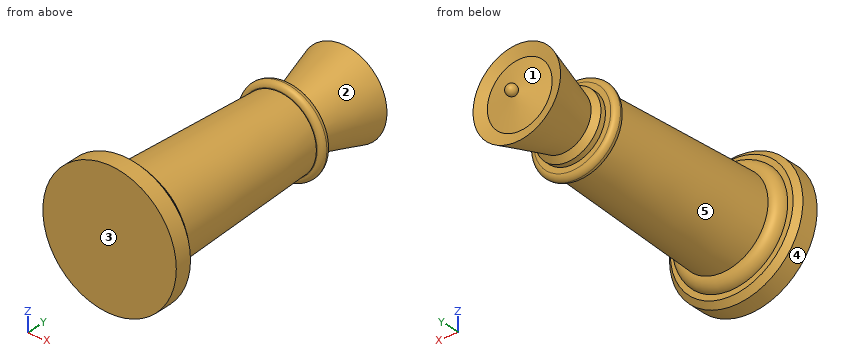
```python
from build123d import *

# Parameters (mm, degrees)
CHAMFER1_SIZE = 0.03
FILLET1_R     = 0.06
FILLET2_R     = 0.03


# Read off the part's stored shape, not the designer's step: Scale1
with BuildPart() as part:
    # Sketch1 → Revolve1 (revolve)
    with BuildSketch(Plane.XY, mode=Mode.PRIVATE) as revolve1_sk:
        with BuildLine():
            Line((0, 0), (-0.375, 0))
            Line((-0.375, 0), (-0.375, 0.125))
            Line((-0.375, 0.125), (-0.315, 0.125))
            Line((-0.315, 0.125), (-0.315, 0.185))
            Line((-0.315, 0.185), (-0.255, 0.185))
            Line((-0.255, 0.185), (-0.212, 1.129))
            Line((-0.212, 1.129), (-0.246, 1.129))
            Line((-0.246, 1.129), (-0.246, 1.189))
            Line((-0.246, 1.189), (-0.186, 1.189))
            Line((-0.186, 1.189), (-0.186, 1.249))
            Line((-0.186, 1.249), (-0.156, 1.249))
            Line((-0.156, 1.249), (-0.246, 1.56))
            Line((-0.246, 1.56), (-0.182, 1.54))
            Line((-0.182, 1.54), (-0.022424467, 1.575071546))
            ThreePointArc((-0.022424467, 1.575071546), (-0.027366527, 1.607291183), (0, 1.625))
            Line((0, 1.625), (0, 0))
        make_face()
    revolve(revolve1_sk.sketch.rotate(Axis((0, 0, 0), (0, 1, 0)), 270), axis=Axis((0, 0, 0), (0, 1, 0)))

    # Chamfer1
    chamfer1_edges = [part.edges().sort_by_distance(p)[0] for p in [
        (0, 0.125, 0.375),
        (0, 1.249, 0.186),
    ]]
    chamfer(chamfer1_edges, length=CHAMFER1_SIZE - 0.0001)  # a hair under: the kernel refuses the full size

    # Fillet1
    fillet1_edges = [part.edges().sort_by_distance(p)[0] for p in [
        (0, 0.185, 0.315),
    ]]
    fillet(fillet1_edges, radius=FILLET1_R - 0.0001)  # a hair under: the kernel refuses the full size

    # Fillet2
    fillet2_edges = [part.edges().sort_by_distance(p)[0] for p in [
        (0, 1.129, 0.246),
        (0, 1.189, 0.246),
    ]]
    fillet(fillet2_edges, radius=FILLET2_R - 0.0001)  # a hair under: the kernel refuses the full size

    # Scale1 outline → Scale1 (revolve)
    with BuildSketch(Plane.XY):
        with BuildLine():
            Line((5.46, 27.865595941), (0.672734004, 28.917742313))
            ThreePointArc((0.672734004, 28.917742313), (0.820995818, 29.884331439), (0, 30.415595941))
            Line((0, 30.415595941), (0, 1.625))
            ThreePointArc((0, 1.625), (0.027366527, 1.607291183), (0.022424467, 1.575071546))
            Line((0.022424467, 1.575071546), (0.182, 1.54))
            Line((0.182, 1.54), (0.246, 1.56))
            Line((0.246, 1.56), (0.156, 1.249))
            Line((0.156, 1.249), (0.186, 1.219))
            Line((0.186, 1.219), (0.186, 1.189))
            Line((0.186, 1.189), (0.216, 1.189))
            ThreePointArc((0.216, 1.189), (0.237213203, 1.180213203), (0.246, 1.159))
            ThreePointArc((0.246, 1.159), (0.237213203, 1.137786797), (0.216, 1.129))
            Line((0.216, 1.129), (0.212, 1.129))
            Line((0.212, 1.129), (0.255, 0.185))
            ThreePointArc((0.255, 0.185), (0.297426407, 0.167426407), (0.315, 0.125))
            Line((0.315, 0.125), (0.345, 0.125))
            Line((0.345, 0.125), (0.375, 0.095))
            Line((0.375, 0.095), (0.375, 0))
            Line((0.375, 0), (0, 0))
            Line((0, 0), (0, -18.334404059))
            Line((0, -18.334404059), (11.25, -18.334404059))
            Line((11.25, -18.334404059), (11.25, -15.484404059))
            Line((11.25, -15.484404059), (10.35, -14.584404059))
            Line((10.35, -14.584404059), (9.45, -14.584404059))
            ThreePointArc((9.45, -14.584404059), (8.922792206, -13.311611853), (7.65, -12.784404059))
            Line((7.65, -12.784404059), (6.36, 15.535595941))
            Line((6.36, 15.535595941), (6.48, 15.535595941))
            ThreePointArc((6.48, 15.535595941), (7.116396103, 15.799199838), (7.38, 16.435595941))
            ThreePointArc((7.38, 16.435595941), (7.116396103, 17.071992044), (6.48, 17.335595941))
            Line((6.48, 17.335595941), (5.58, 17.335595941))
            Line((5.58, 17.335595941), (5.58, 18.235595941))
            Line((5.58, 18.235595941), (4.68, 19.135595941))
            Line((4.68, 19.135595941), (7.38, 28.465595941))
            Line((7.38, 28.465595941), (5.46, 27.865595941))
        make_face()
    revolve(axis=Axis((0, 0, 0), (0, 1, 0)))


solid = part.part
```
Here's how the part is built. I have some questions about the finished solid (model axes, mm). Face numbers are marked on the shaded views. A direction names the side the tool comes from. Give positions to 0.01 mm unless a question says otherwise; leave off trailing zeros. Order: outer loops, then holes, each group sorted by start corner. A loop starts at its lowest first (then second) coordinate and runs counter-clockwise, first axis right, second up. Notation, with made-up numbers: (71, 8.5) -> (81, 8.5) arc R24 ccw to (81, 46.5) -> close; hole circle Ø5 at (-40, 6). An arc over 180 degrees is marked (long way). Use CSV: the item, a comma, the result in double quotes. Start each with the question number.
Item 1: If I drill on probe 1 along Y at (x, z) = (9.25, 3.5); probe 2 along X at (y, z) = (-0.5, -5); probe 3 along X at (y, z) = (14, -2), over which ranges is the centre line in solid material (lowest first)? Write a range as [from, to].
Item 2: Thinking about a two-plate mould opening in X: for the marked faces 1, 2 and 3, which applies, pulls with the +X half, pulls with the -X half, needs draft (parallel to the pull), parting line crosses it, or undercut?
Item 3: On a 3-axis mill with a long thin cutter (end or side, diameter ignored), from which of +Z, -Z, +X, -X, +Y, -Y can I reach the whole of each face in a straight line? I mean the marked faces 4 and 5. Say none if no direction works.
Item 4: I'm going to push flat-ended pins straight in: P1, Ø4, axis at x = -2.5, z = -2, coming from the +Y side; P2, Ø10, axis at x = 6.5, z = -2.5, coming from the +Y side; P3, Ø1.5, axis at x = 1, y = 9, coming from the +Z side. Where does each tip first touch, or does it pass through?
Item 5: Suppose I cut it at A-A (y = 8). List the corners of the cut face in (x, z) for me.
Item 6: Suppose I cut it at B-B (y = -1.5). List the corners of the cut face in (x, z) for me.
Answer block:
1,probe 1,"y = [-18.33, -14.58]"
1,probe 2,"x = [-5.03, 5.03]"
1,probe 3,"x = [-6.11, 6.11]"
2,face 1,"undercut"
2,face 2,"parting line crosses it"
2,face 3,"needs draft"
3,face 4,"+Y, -Y"
3,face 5,"none"
4,P1,"stops at y = 28.8"
4,P2,"stops at y = 28.63"
4,P3,"stops at z = 6.67"
5,outline,"circle Ø13.41 at (0, 0)"
6,outline,"circle Ø14.27 at (0, 0)"
